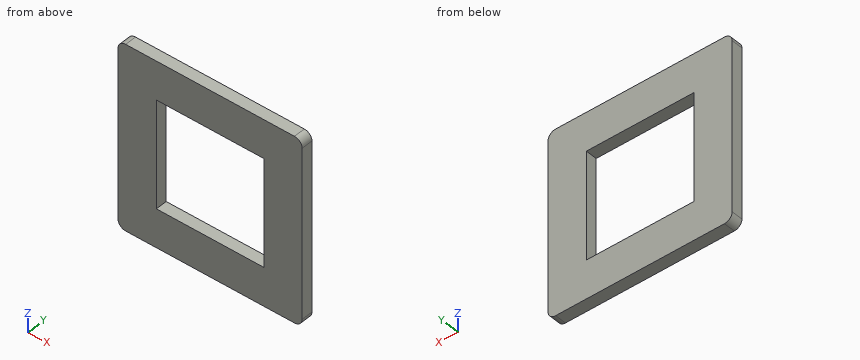
from build123d import *

# Parameters (mm, degrees)
SKETCH_1_W      = 24
SKETCH_1_H      = 24
SKETCH_1_W_2    = 14
SKETCH_1_H_2    = 14
EXTRUDE_1_DEPTH = 1.5
FILLET_1_R      = 1


with BuildPart() as part:
    # 草图1 → 凸台-拉伸1 (new body)
    with BuildSketch(Plane(origin=(0, 0, 0), x_dir=(1, 0, 0), z_dir=(0, 1, 0))):
        Rectangle(SKETCH_1_W, SKETCH_1_H)
        Rectangle(SKETCH_1_W_2, SKETCH_1_H_2, mode=Mode.SUBTRACT)
    extrude(amount=EXTRUDE_1_DEPTH)

    # 圆角1
    fillet_1_edges = [part.edges().sort_by_distance(p)[0] for p in [
        (-12, 0.75, 12),
        (-12, 0.75, -12),
        (12, 0.75, -12),
        (12, 0.75, 12),
    ]]
    fillet(fillet_1_edges, radius=FILLET_1_R)


solid = part.part
CAD build for the part. Positions are in the model's coordinates, mm. Give positions to 0.01 mm unless a question says otherwise; leave off trailing zeros. Write each loop counter-clockwise with the first axis right and the second up, starting at its lowest first coordinate (ties: lowest second). Pieces come first, ordered by that corner, then holes. Notation, with made-up numbers: (46.5, 9.25) -> (90.5, 9.25) arc R15 ccw to (90.5, 27.25) -> close; hole circle Ø11 at (6, 16.5). An arc over 180 degrees is marked (long way). Return JSON: item names as keys, results as strings.
Item 1: Drill centre line: probe 1 along X at (y, z) = (1.2, -0.5). Where is it in solid material? Low to high.
Answer below:
{"probe 1": "x = -12 to -7, 7 to 12"}
Item 2: Band-saw the part on A-A (x = 4.5). List the corners of the cut face in (y, z).
Answer below:
{"outline": "(0, -12) -> (1.5, -12) -> (1.5, -7) -> (0, -7) -> close; (0, 7) -> (1.5, 7) -> (1.5, 12) -> (0, 12) -> close"}
Item 3: Band-saw the part on C-C (z = 1.25). List the corners of the cut face in (x, y), then the cut area to 3 significant figures.
Answer below:
{"outline": "(-12, 0) -> (-7, 0) -> (-7, 1.5) -> (-12, 1.5) -> close; (7, 0) -> (12, 0) -> (12, 1.5) -> (7, 1.5) -> close", "area": "15.0 mm2"}
Item 4: Band-saw the part on B-B (y = 0.65). List the corners of the cut face in (x, z).
Answer below:
{"outline": "(-12, -11) arc R1 ccw to (-11, -12) -> (11, -12) arc R1 ccw to (12, -11) -> (12, 11) arc R1 ccw to (11, 12) -> (-11, 12) arc R1 ccw to (-12, 11) -> close; hole (-7, -7) -> (7, -7) -> (7, 7) -> (-7, 7) -> close"}
